```python
from build123d import *

# Parameters (mm, degrees)
PAD001_DEPTH    = 1
PAD008_DEPTH    = 1
SKETCH028_R     = 1.144433
POCKET014_DEPTH = 1


with BuildPart() as part:
    # Sketch013 → Pad001 (new body)
    with BuildSketch(Plane(origin=(0, 0, 1), x_dir=(1, 0, 0), z_dir=(0, 0, -1))):
        with BuildLine():
            Line((-43.791128, 29.5), (41.9, 29.5))
            ThreePointArc((44.5, 26.9), (43.738478, 28.738478), (41.9, 29.5))
            Line((44.5, 26.9), (44.5, -8))
            Line((44.5, -8), (44.5, -26.9))
            ThreePointArc((41.9, -29.5), (43.738478, -28.738478), (44.5, -26.9))
            Line((41.9, -29.5), (-43.993837, -29.5))
            ThreePointArc((-44.7, -28.066977), (-44.427413, -28.823154), (-43.993837, -29.5))
            Line((-44.7, -28.066977), (-44.7, 27.986088))
            ThreePointArc((-43.791128, 29.5), (-44.339824, 28.799633), (-44.7, 27.986088))
        make_face()
    extrude(amount=-PAD001_DEPTH)

    # Sketch (on Face8 of Pad001) → Pad008 (join)
    with BuildSketch(Plane(origin=(0, 0, 1), x_dir=(1, 0, 0), z_dir=(0, 0, -1))):
        with BuildLine():
            Line((-42.5, 28.5), (41.5, 28.5))
            ThreePointArc((43.5, 26.5), (42.914214, 27.914214), (41.5, 28.5))
            Line((43.5, 26.5), (43.5, -26.5))
            ThreePointArc((41.5, -28.5), (42.914214, -27.914214), (43.5, -26.5))
            Line((41.5, -28.5), (-42.5, -28.5))
            ThreePointArc((-44.5, -26.5), (-43.914214, -27.914214), (-42.5, -28.5))
            Line((-44.5, -26.5), (-44.5, 26.5))
            ThreePointArc((-42.5, 28.5), (-43.914214, 27.914214), (-44.5, 26.5))
        make_face()
    extrude(amount=PAD008_DEPTH)

    # Sketch028 (on Face19 of Pad008) → Pocket014 (cut)
    with BuildSketch(Plane(origin=(0, 0, 0), x_dir=(1, 0, 0), z_dir=(0, 0, -1))):
        with BuildLine():
            ThreePointArc((-28.239604, 20.682525), (-36.772568, -0.055356), (-28.16139, -20.760883))
            ThreePointArc((-31.495352, -24.403687), (-28.034523, -24.224048), (-28.16139, -20.760883))
            ThreePointArc((-31.441869, 24.45629), (-41.706794, 0.037508), (-31.495352, -24.403687))
            ThreePointArc((-28.239604, 20.682525), (-28.010921, 24.122116), (-31.441869, 24.45629))
        make_face()
        with BuildLine():
            ThreePointArc((-20.815283, 15.021339), (-27.551042, 0.307322), (-21.268036, -14.605646))
            ThreePointArc((-24.552994, -17.595228), (-21.393816, -17.766988), (-21.268036, -14.605646))
            ThreePointArc((-24.215721, 17.808685), (-31.954171, 0.178842), (-24.552994, -17.595228))
            ThreePointArc((-20.815283, 15.021339), (-21.261111, 17.945313), (-24.215721, 17.808685))
        make_face()
        with BuildLine():
            ThreePointArc((-13.536319, 7.856117), (-17.438434, 0.075734), (-13.740768, -7.803868))
            ThreePointArc((-16.96495, -11.074563), (-13.821902, -10.948401), (-13.740768, -7.803868))
            ThreePointArc((-16.837212, 11.183151), (-22.04722, 0.083828), (-16.96495, -11.074563))
            ThreePointArc((-13.536319, 7.856117), (-13.584742, 11.10907), (-16.837212, 11.183151))
        make_face()
        with BuildLine():
            ThreePointArc((4.243843, 18.27707), (-4.248678, 23.579205), (-10.782384, 15.993281))
            Line((-10.782384, 15.993281), (-10.782384, -13.42268))
            ThreePointArc((-10.782384, -13.42268), (-1.89675, -23.128113), (7.426263, -13.842029))
            ThreePointArc((7.426263, -13.842029), (19.95175, -3.341626), (11.392084, 10.582396))
            ThreePointArc((11.392084, 10.582396), (10.373826, 16.804092), (4.243843, 18.27707))
        make_face()
        with Locations((-4.272868, 13.992623)):
            Circle(SKETCH028_R, mode=Mode.SUBTRACT)
        with BuildLine():
            ThreePointArc((2.411883, 6.249422), (0.960031, 9.950894), (-2.428904, 12.030293))
            ThreePointArc((-1.741453, 13.60297), (-2.704463, 13.087334), (-2.428904, 12.030293))
            ThreePointArc((4.082151, 6.635487), (2.262958, 11.03246), (-1.741453, 13.60297))
            ThreePointArc((2.411883, 6.249422), (3.441947, 5.599114), (4.082151, 6.635487))
        make_face(mode=Mode.SUBTRACT)
    extrude(amount=-POCKET014_DEPTH, mode=Mode.SUBTRACT)


solid = part.part
```
Part model, mm, in its own coordinate system. A direction names the side the tool comes from. Give positions to 0.01 mm unless a question says otherwise; leave off trailing zeros. Order: outer loops, then holes, each group sorted by start corner. A loop starts at its lowest first (then second) coordinate and runs counter-clockwise, first axis right, second up. Notation, with made-up numbers: M 53.5,-39.5 L 64.5,-39.5 A19 cw 64.5,-34.5 Z; hole C 34.5,2 d7. An arc over 180 degrees is marked long. Use a Markdown table: item, result. Add a question column.
(1) Probe line 1 along X through (y, z) = (10.5, 0.8) (3 decimals); line 2 along X through (y, z) = (5, 0.3); line 3 along X through (y, z) = (-22.5, 0.15). List the from-to ranges inside material, lowest first. Write a range as [from, to].
(2) Drop flat-ended pins along their axis: P1, Ø0.5, axis at x = 16, z = 0.5, coming from the -Y side; P2, Ø0.8, axis at y = -6, z = 0.5, coming from the +X side. Give the stop position or say it passes through.
(3) Mould opens along X. For faces 5 (the face through (-22.045, -0.261, 0.493)), 6 (the face through (-13.856, 10.983, 0.493)), 7 (the face through (0, -29, 1)), 8 (the face through (42.93, -27.9, 0.51)) say: +X half, -X half, draft (parallel to the pull), parting line (faces both ways), or undercut.
(4) Saw through at A-A, the plane z = 0.7. Give the number of separate pieces and of enclosed holes in the cut face, and give its area (3 significant figures).
(5) Saw through at D-D, the plane x = 15. Give the cut face in (y, z).
(6) Saw through at C-C, the plane y = 2.5. Give the cut face in (x, z).
(7) Saw through at B-B, the plane x = 34. Give the cut face in (y, z), and give its area (3 significant figures).
(8) 3-axis set-ups, long thin cutter, end or side, ignore diameter. For faces 1 (the face through (-43.93, 27.9, 0.51)), 2 (the face through (43.718, 28.759, 1.493)), 3 (the face through (-43.9, -27.93, 0.51)), 4 (the face through (-28.07, 24.26, 0.49)): which of +Z, -Z, +X, -X, +Y, -Y reach the whole face in a straight line?
Answer key:
| question | item | result |
|---|---|---|
| 1 | line 1 | [-44.5, -40.058], [-34.829, -29.615], [-24.595, -17.595], [-13.477, -10.782], [16.119, 43.5] |
| 1 | line 2 | [-44.5, -41.34], [-36.34, -31.45], [-26.92, -21.17], [-16.13, -10.78], [19.57, 43.5] |
| 1 | line 3 | [-44.5, -33.28], [-27.42, -7.16], [0.98, 43.5] |
| 2 | P1 | y = -28.5 |
| 2 | P2 | x = 43.5 |
| 3 | face 5 | undercut |
| 3 | face 6 | undercut |
| 3 | face 7 | draft |
| 3 | face 8 | +X half |
| 4 | separate pieces | 3 |
| 4 | enclosed holes | 4 |
| 4 | area | 3,420 mm^2 |
| 5 | outline | M -29.5,1 L -28.5,1 L -28.5,0 L -8.75,0 L -8.75,1 L 11.42,1 L 11.42,0 L 28.5,0 L 28.5,1 L 29.5,1 L 29.5,2 L -29.5,2 Z |
| 6 | outline | M -44.7,1 L -44.5,1 L -44.5,0 L -41.62,0 L -41.62,1 L -36.67,1 L -36.67,0 L -31.83,0 L -31.83,1 L -27.4,1 L -27.4,0 L -21.83,0 L -21.83,1 L -17.13,1 L -17.13,0 L -10.78,0 L -10.78,1 L 20.06,1 L 20.06,0 L 43.5,0 L 43.5,1 L 44.5,1 L 44.5,2 L -44.7,2 Z |
| 7 | outline | M -29.5,1 L -28.5,1 L -28.5,0 L 28.5,0 L 28.5,1 L 29.5,1 L 29.5,2 L -29.5,2 Z |
| 7 | area | 116 mm^2 |
| 8 | face 1 | -Z, -X, +Y |
| 8 | face 2 | +Z, -Z, +X, +Y |
| 8 | face 3 | -Z, -X, -Y |
| 8 | face 4 | -Z |
